Verification items for this drawing (mm, ordinates from the low corner). A direction names the side the tool comes from. Coordinates: 2 decimals unless noted, no trailing zeros. Order: outer loops, then holes, each group sorted by start corner. A loop starts at its lowest first (then second) coordinate and runs counter-clockwise, first axis right, second up.
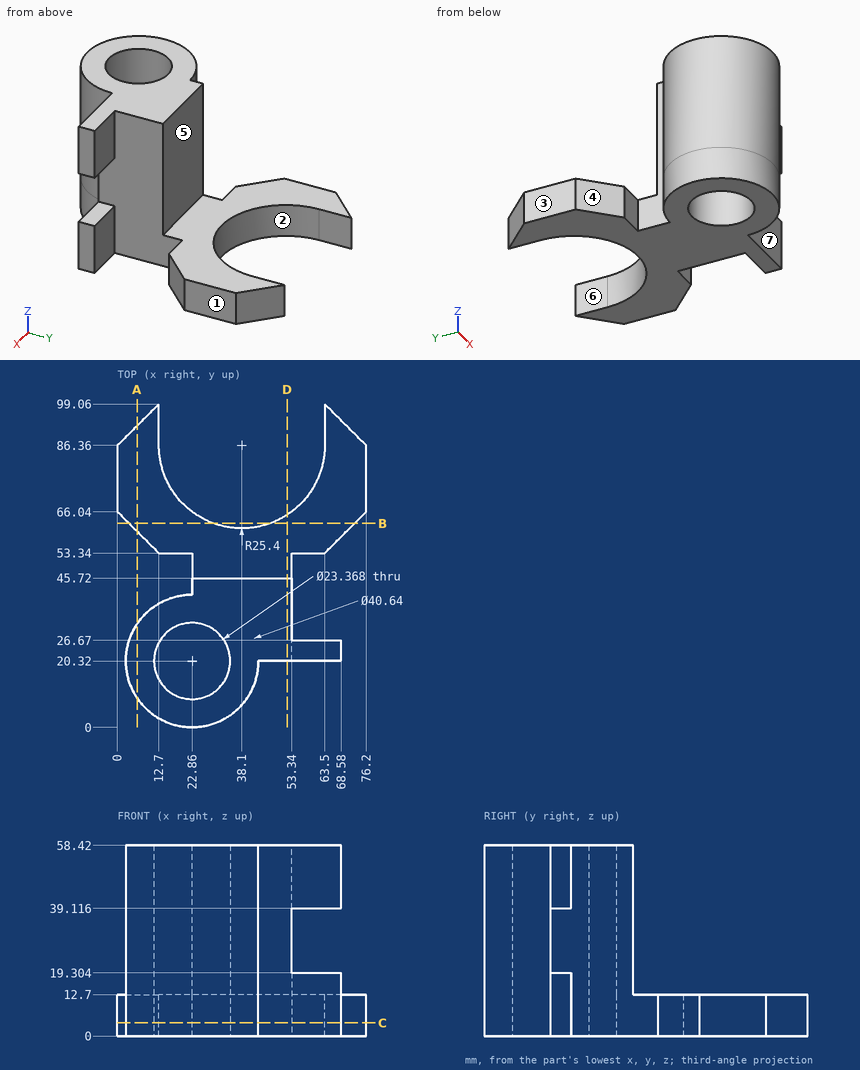
(1) Cross-section at A-A (x = 6). Enter the section's corners in (y, z).
Filled in:
outline: (8.98, 0) - (31.66, 0) - (31.66, 58.42) - (8.98, 58.42) - close; (60.04, 0) - (92.36, 0) - (92.36, 12.7) - (60.04, 12.7) - close
(2) Tool access check on the marked faces 4, 5, 6 and 7. Record the directions out of +Z, -Z, +X, -X, +Y, -Y that give a thin tool (end or side, any length) a straight path to the whole face; none if there is none.
Filled in:
face 4: +Z, -Z, -X
face 5: +Z, +X, -X, +Y
face 6: +Z, -Z, +Y
face 7: +Z, -Z, +X, -Y
(3) Cross-section at B-B (y = 62.5). Enter the section's corners in (x, z), and give its area (3 significant figures).
Filled in:
outline: (3.54, 0) - (29.39, 0) - (29.39, 12.7) - (3.54, 12.7) - close; (46.81, 0) - (72.66, 0) - (72.66, 12.7) - (46.81, 12.7) - close
area: 657 mm2
(4) Thickness scan on probe 1 along Y at (x, z) = (19, 11); probe 2 along Y at (x, z) = (66.5, 42.5); probe 3 along X at (y, z) = (20, 42). Record the ranges inside material, lowest first.
Filled in:
probe 1: y = 0.37 to 9.29, 31.35 to 40.27, 53.34 to 69.62
probe 2: y = 20.32 to 26.67
probe 3: x = 2.54 to 11.18, 34.54 to 43.18
(5) Cross-section at C-C (z = 4). Enter the section's corners in (x, y), and give its area (3 significant figures).
Filled in:
outline: (0, 66.04) - (12.7, 53.34) - (22.86, 53.34) - (22.86, 40.64) arc R20.32 ccw (long way) to (43.18, 20.32) - (68.58, 20.32) - (68.58, 26.67) - (53.34, 26.67) - (53.34, 53.34) - (63.5, 53.34) - (76.2, 66.04) - (76.2, 86.36) - (63.5, 99.06) - (63.5, 86.36) arc R25.4 cw to (12.7, 86.36) - (12.7, 99.06) - (0, 86.36) - close; hole circle Ø23.37 at (22.86, 20.32)
area: 3,150 mm2
(6) Go/stop test with flat-tipped pins: P1, Ø3, axis at x = 16, z = 6.5, coming from the -Y side; P2, Ø14, axis at x = 22.86, y = 20.32, coming from the +Z side; P3, Ø4, axis at y = 94, z = 3.5, coming from the +X side; P4, Ø3, axis at x = 56.5, z = 9.5, coming from the -Y side. Record where each tip stops, or that it passes through.
Filled in:
P1: stops at y = 0.72
P2: passes through
P3: stops at x = 70.56
P4: stops at y = 20.32
(7) Cross-section at D-D (x = 52). Enter the section's corners in (y, z).
Filled in:
outline: (20.32, 0) - (65.1, 0) - (65.1, 12.7) - (45.72, 12.7) - (45.72, 58.42) - (20.32, 58.42) - close
(8) Release check for a two-part mould opening along X. For the marked faces 1, 2 and 3 record: +X half, -X half, draft (parallel to the pull), parting line (faces both ways), or undercut.
Filled in:
face 1: +X half
face 2: undercut
face 3: -X half
